from build123d import *

# Parameters (mm, degrees)
SKETCH_W          = 57.15
SKETCH_H          = 20.32
SKETCH_R          = 1.651
PAD_DEPTH         = 3.175
SKETCH001_R       = 1.905
PAD001_DEPTH      = 15.175
SKETCH002_R       = 0.9525
POCKET_DEPTH      = 15.875
PAD002_DEPTH      = 15.24
PAD002_DEPTH_BACK = 5.1402
FILLET_R          = 1.27
CHAMFER_SIZE      = 12.7
CHAMFER001_SIZE   = 3.048
SKETCH004_R       = 3.2131
POCKET001_DEPTH   = 3.81762
SKETCH005_W       = 23.563626
SKETCH005_H       = 25.4
PAD003_DEPTH      = 1.5875
FILLET001_R       = 3.175


with BuildPart() as ball1:
    # Sphere → Sphere (revolve)
    with BuildSketch(Plane(origin=(34.925, 11.16, 19.304), x_dir=(1, 0, 0), z_dir=(0, -1, 0))):
        with BuildLine():
            ThreePointArc((0, -1.5875), (1.5875, 0), (0, 1.5875))
            Line((0, 1.5875), (0, -1.5875))
        make_face()
    revolve(axis=Axis((34.925, 11.16, 19.304), (0, 0, 1)))


with BuildPart() as ball002:
    # Sphere001 → Sphere001 (revolve)
    with BuildSketch(Plane(origin=(22.225, 11.16, 19.304), x_dir=(1, 0, 0), z_dir=(0, -1, 0))):
        with BuildLine():
            ThreePointArc((0, -1.5875), (1.5875, 0), (0, 1.5875))
            Line((0, 1.5875), (0, -1.5875))
        make_face()
    revolve(axis=Axis((22.225, 11.16, 19.304), (0, 0, 1)))


with BuildPart() as fusion:
    # Sketch → Pad (new body, symmetric)
    with BuildSketch(Plane.XY):
        with Locations((28.575, 10.16)):
            Rectangle(SKETCH_W, SKETCH_H)
        with Locations((6.731, 10.16)):
            Circle(SKETCH_R, mode=Mode.SUBTRACT)
        with Locations((50.419, 10.16)):
            Circle(SKETCH_R, mode=Mode.SUBTRACT)
    extrude(amount=PAD_DEPTH, both=True)

    # Sketch001 (on Face8 of Pad) → Pad001 (join)
    with BuildSketch(Plane.XY.offset(3.175)):
        with Locations((22.225, 11.16)):
            Circle(SKETCH001_R)
        with Locations((34.925, 11.16)):
            Circle(SKETCH001_R)
    extrude(amount=PAD001_DEPTH)

    # Sketch002 (on Face4 of Pad001) → Pocket (cut)
    with BuildSketch(Plane(origin=(0, 0, -3.175), x_dir=(1, 0, 0), z_dir=(0, 0, -1))):
        with Locations((22.225, -11.16)):
            Circle(SKETCH002_R)
        with Locations((34.925, -11.16)):
            Circle(SKETCH002_R)
    extrude(amount=-POCKET_DEPTH, mode=Mode.SUBTRACT)

    # Sketch003 (on Face6 of Pocket) → Pad002 (join, two sides)
    with BuildSketch(Plane.XZ) as pad002_sk:
        Polygon((40.356813, 3.175), (40.356813, 22.711586), (21.857486, 4.212258), (19.612422, 6.457322), (19.612422, 3.175), align=None)
    extrude(amount=PAD002_DEPTH)
    extrude(pad002_sk.sketch, amount=-PAD002_DEPTH_BACK)

    # Fillet
    fillet_edges = [fusion.edges().sort_by_distance(p)[0] for p in [
        (33.9725, 11.16, -3.175),
        (21.2725, 11.16, -3.175),
    ]]
    fillet(fillet_edges, radius=FILLET_R)

    # Chamfer
    chamfer_edges = [fusion.edges().sort_by_distance(p)[0] for p in [
        (40.356813, -7.62, 3.175),
    ]]
    chamfer(chamfer_edges, length=CHAMFER_SIZE)

    # Chamfer001
    chamfer001_edges = [fusion.edges().sort_by_distance(p)[0] for p in [
        (23.634617, 0, 3.175),
    ]]
    chamfer(chamfer001_edges, length=CHAMFER001_SIZE)

    # Sketch004 (on Face2 of Chamfer001) → Pocket001 (cut)
    with BuildSketch(Plane(origin=(12.240907, 0, -12.240907), x_dir=(0, 1, 0), z_dir=(0.707107, 0, -0.707107))):
        with Locations((-10.16, 26.67)):
            Circle(SKETCH004_R)
        with Locations((-5.08, 34.29)):
            Circle(SKETCH004_R)
    extrude(amount=-POCKET001_DEPTH, mode=Mode.SUBTRACT)

    # Sketch005 (on Face15 of Pocket001) → Pad003 (join)
    with BuildSketch(Plane(origin=(0, 5.1402, 0), x_dir=(-1, 0, 0), z_dir=(0, 1, 0))):
        with Locations((-28.575, 15.875)):
            Rectangle(SKETCH005_W, SKETCH005_H)
    extrude(amount=PAD003_DEPTH)

    # Fillet001
    fillet001_edges = [fusion.edges().sort_by_distance(p)[0] for p in [
        (40.356813, 5.93395, 28.575),
        (16.793187, 5.93395, 28.575),
    ]]
    fillet(fillet001_edges, radius=FILLET001_R)

    # Fusion: union Ball1, Ball002
    add(ball1.part)
    add(ball002.part)


solid = fusion.part
Input: part model. Units: mm. Frame: model coordinates. A direction names the side the tool comes from. Give positions to 0.01 mm unless a question says otherwise; leave off trailing zeros. Write each loop counter-clockwise with the first axis right and the second up, starting at its lowest first coordinate (ties: lowest second). Pieces come first, ordered by that corner, then holes.
Q1. Material intervals for probe 1 along X at (y, z) = (10, -1); probe 2 along Y at (x, z) = (11.5, 0); probe 3 along Z at (x, y) = (3.5, 6) (3 decimals), sorted ascending.
Q2. Set-up query: faces 4 (the face through (24, -9, 3.175)), 5 (the face through (34.34, -7.51, 9.86)), 6 (the face through (16.793, 6, 14)), 7 (the face through (22.02, 12.09, 5.3)), 8 (the face through (20.32, 11.24, 10.66)). Return all of +Z, -Z, +X, -X, +Y, -Y with unobstructed straight access to the full face (end or side cutting, diameter ignored); none if empty.
Q3. Section C-C, the plane x = 16. Output: boundary loops of the cut face in (y, z) (3 decimals), plus the area to 3 significant figures.
Q4. Section A-A, the plane z = -1. State how many separate pieces and enclosed holes the cut face has, plus the area to 3 significant figures.
Q5. Pull-direction query (Y, two-part tool) for faces 1 (the face through (31.237, -5.193, 13.591)), 2 (the face through (48.77, 10.23, -0.04)), 3 (the face through (26, 5.14, 19)); classes: pulls with the +Y half, pulls with the -Y half, needs draft (parallel to the pull), parting line crosses it, or undercut.
Q6. First-contact query: P1, Ø0.8, axis at y = 6, z = 18, coming from the -X side; P2, Ø2, axis at x = 37.5, z = 16.5, coming from the +Y side; P3, Ø1.1, axis at x = 22.225, y = 11.16, coming from the +Z side; P4, Ø7, axis at y = 0, z = 2.5, coming from the -X side. Flat tips, straight axial feed; report the tip coordinate or a pass-through.
Q7. Section B-B, the plane y = -9.5. Output: boundary loops of the cut face in (x, z) (3 decimals).
Filled in:
1. probe 1: x = 0 to 5.09, 8.37 to 48.78, 52.06 to 57.15
1. probe 2: y = 0 to 20.32
1. probe 3: z = -3.175 to 3.175
2. face 4: -Z, +X, -X, -Y
2. face 5: -Z, +X, -Y
2. face 6: +Z, -X, +Y, -Y
2. face 7: -Z
2. face 8: +Z
3. outline: (0, -3.175) - (20.32, -3.175) - (20.32, 3.175) - (0, 3.175) - close
3. area: 129 mm2
4. separate pieces: 1
4. enclosed holes: 4
4. area: 1,140 mm2
5. face 1: needs draft
5. face 2: undercut
5. face 3: pulls with the -Y half
6. P1: stops at x = 16.79
6. P2: stops at y = 12.23
6. P3: stops at z = 20.89
6. P4: stops at x = 0
7. outline: (19.612, 3.175) - (27.657, 3.175) - (28.876, 4.394) - (26.176, 7.094) - (30.624, 11.541) - (33.323, 8.841) - (40.357, 15.875) - (40.357, 22.712) - (21.857, 4.212) - (19.612, 6.457) - close
